Here's the drawing with two shaded views (mm, measured from the low corner). I have some questions. Give positions to 0.01 mm unless a question says otherwise; leave off trailing zeros. Write each loop counter-clockwise with the first axis right and the second up, starting at its lowest first coordinate (ties: lowest second). Pieces come first, ordered by that corner, then holes.
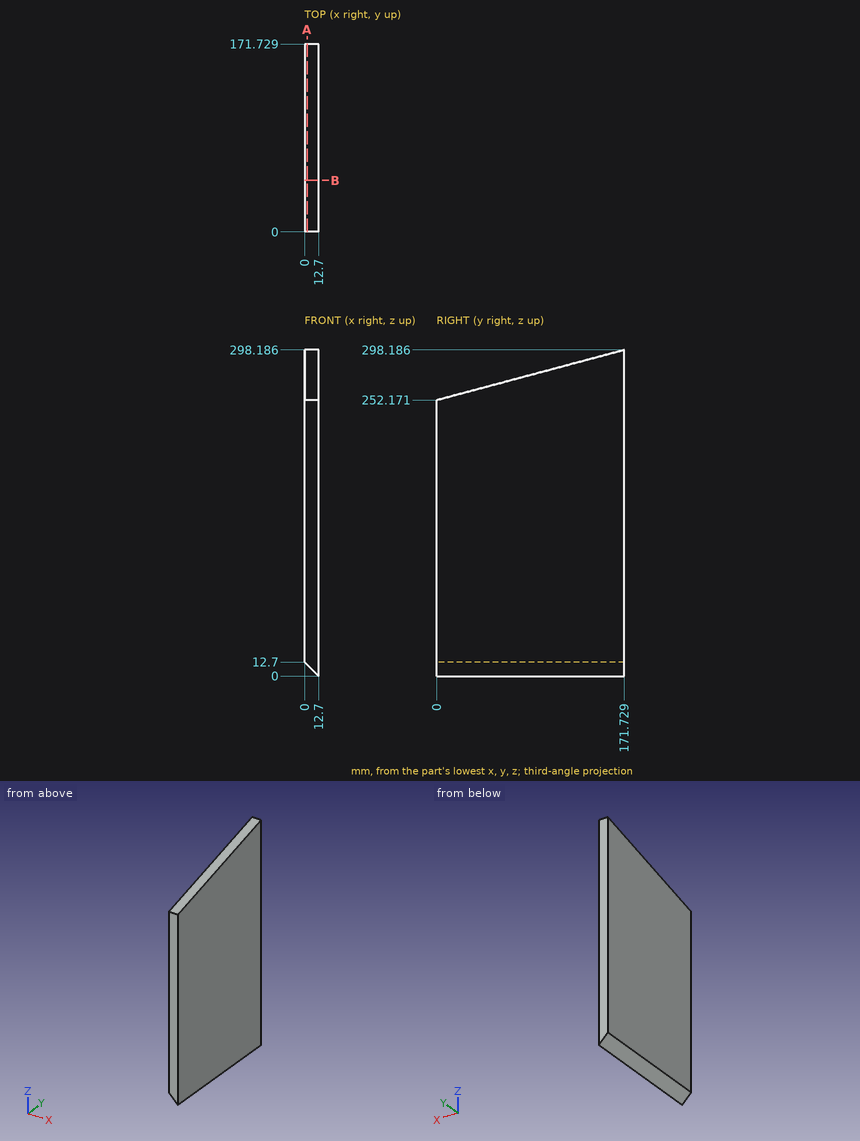
1) Please list where these lines run through material, in increasing order: L1, parallel to Z at x = 8, y = 107.5 (1 decimal); L2, parallel to Z at x = 8.5, y = 139 (1 decimal).
Values follow:
L1: z = 4.7 to 281
L2: z = 4.2 to 289.4
2) For pin 1 Ø3 at (x, y) = (8.5, 38.5) entering from +Z; pin 2 Ø3 at (x, y) = (2, 87) entering from -Z, each with a flat end and sliding along its axis, tell me the tip position at first contact or that it passes through.
Values follow:
pin 1: stops at z = 262.89
pin 2: stops at z = 9.2
3) Suppose I cut it at B-B on y = 47. Write out the boundary of the cut face in (x, z) (1 decimal).
Values follow:
outline: (0, 12.7) - (12.7, 0) - (12.7, 264.8) - (0, 264.8) - close
4) Suppose I cut it at A-A on x = 2.25. Write out the boundary of the cut face in (y, z), plus the area to 3 significant figures.
Values follow:
outline: (0, 10.45) - (171.73, 10.45) - (171.73, 298.19) - (0, 252.17) - close
area: 45,500 mm2
